Autodesk Inventor part; units mm, degrees
ref_plane "YZ Plane" through (0, 0, 0) normal (1, 0, 0) x (0, 1, 0)
ref_plane "XZ Plane" through (0, 0, 0) normal (0, 1, 0) x (-1, 0, 0)
ref_plane "XY Plane" through (0, 0, 0) normal (0, 0, 1) x (1, 0, 0)
sketch "Эскиз1" plane through (0, 0, 0) normal (0, 0, 1) x (1, 0, 0)
  line L0 (0, 0) -> (0, 6.4157)
  line L1 (2.5, 4.85) -> (20, 4.85)
  line L2 (20, 4.85) -> (20, 2.95)
  line L3 (20, 2.95) -> (25, 2.95)
  line L4 (25, 2.95) -> (25, 1.75)
  line L5 (25, 1.75) -> (0, 1.75)
  line L6 (0, 0) -> (17.5335, 0) construction
  line L7 (0, 6.4157) -> (1, 7.5)
  line L8 (1, 7.5) -> (2.5, 7.5)
  line L9 (2.5, 7.5) -> (2.5, 4.85)
  dimension "d0" = 5.9
  dimension "d2" = 3.5
  dimension "d3" = 9.7
  dimension "d12" = 15
  dimension "d18" = 1
  dimension "d19" = 5
  dimension "d21" = 2.5
  dimension "d22" = 17.5
revolve "Вращение1" add sketch "Эскиз1" angle 360 about axis through (0, 0, 0) along (1, 0, 0)
chamfer "Фаска1" distance 0.5 angle 45 2 edges at (20, -4.85, 0) (0, -1.75, 0)
chamfer "Фаска2" distance 0.1 angle 45 2 edges at (25, -2.95, 0) (25, -1.75, 0)
properties part number "Ось односторонняя"
Input: part model. Units: mm. Frame: model coordinates. A direction names the side the tool comes from. Coordinates: 2 decimals unless noted, no trailing zeros. Loops run counter-clockwise (first coordinate to the right, second up) from the corner with the lowest first, then second, coordinate; pieces in that order, holes last. Notation, with made-up numbers: M 13.25,14 L 60.25,14 A12 cw 60.25,32 Z; hole C 71.25,11.5 d5. An arc over 180 degrees is marked long. One line per item, written item: value.
(1) Pull-direction query (Z, two-part tool) for faces 3 (the flat face through (25, 1, -2)), 4 (the cylindrical face through (12.529, 1.617, 0.67)), 5 (the cylindrical face through (22.484, -2.947, 0.13)); classes: +Z half, -Z half, draft (parallel to the pull), parting line (faces both ways), or undercut.
Filled in:
face 3: draft
face 4: undercut
face 5: parting line
(2) Section A-A (y = 0). Output: boundary loops of the cut face in (x, z), and give its area (3 significant figures).
Filled in:
outline: M 0,-6.42 L 1,-7.5 L 2.5,-7.5 L 2.5,-4.85 L 19.5,-4.85 L 20,-4.35 L 20,-2.95 L 24.9,-2.95 L 25,-2.85 L 25,-1.85 L 24.9,-1.75 L 0.5,-1.75 L 0,-2.25 Z; M 0,2.25 L 0.5,1.75 L 24.9,1.75 L 25,1.85 L 25,2.85 L 24.9,2.95 L 20,2.95 L 20,4.35 L 19.5,4.85 L 2.5,4.85 L 2.5,7.5 L 1,7.5 L 0,6.42 Z
area: 148 mm^2
(3) Line query: line 1 along Z through (x, y) = (7.5, 0); line 2 along X through (y, z) = (2.5, -5.75); line 3 along X through (y, z) = (2.5, -3.5). Output: solid intervals per line, ascending. Write a range as from..to.
Filled in:
line 1: -4.85..-1.75, 1.75..4.85
line 2: 0..2.5
line 3: 0..20
(4) Pin query (flat end, axial travel): pin 1 (8 mm diameter, centred on x = 11, z = -3.5, fed in from -Y); pin 2 (8 mm diameter, centred on x = 10.5, y = -4.5, fed in from +Z); pin 3 (6 mm diameter, centred on y = -5, z = 2, fed in from -X); pin 4 (1.5 mm diameter, centred on x = 4.5, y = -3.5, fed in from -Z) (3 decimals). Return the tip coordinate at first contact, or that it passes through.
Filled in:
pin 1: y = -4.85
pin 2: z = 4.82
pin 3: x = 0
pin 4: z = -3.995
(5) Section C-C (x = 6.5). Output: boundary loops of the cut face in (y, z), and give its area (3 significant figures).
Filled in:
outline: C 0,0 d9.7; hole C 0,0 d3.5
area: 64.3 mm^2
(6) Reachability of faces 1 (the flat face through (20, 3, -1)), 2 (the flat face through (0, 0, -3)) from +Z, -Z, +X, -X, +Y, -Y: full face, straight path, thin tool, end or side. Return the list, or none.
Filled in:
face 1: +X
face 2: +Z, -Z, -X, +Y, -Y
